```python
from build123d import *

# Parameters (mm, degrees)
BASPROSKE_W        = 5
BASPROSKE_H        = 7
TOOTHCUT_DEPTH     = 12.090536506
TEETHCUTS_COUNT    = 12
TEETHCUTS_ANGLE    = 330
BORSKE_R           = 2.5
BORE_DEPTH         = 50.0000508
SKETCH1_W          = 20.08971131
SKETCH1_H          = 17.337649252
CUT_EXTRUDE3_DEPTH = 0.25


with BuildPart() as part:
    # BasProSke → Base-Revolve (revolve)
    with BuildSketch(Plane(origin=(0, 0, 0), x_dir=(1, 0, 0), z_dir=(0, 1, 0)), mode=Mode.PRIVATE) as base_revolve_sk:
        with Locations((2.5, 3.5)):
            Rectangle(BASPROSKE_W, BASPROSKE_H)
    revolve(base_revolve_sk.sketch.rotate(Axis((-10, 0, 0), (1, 0, 0)), 180), axis=Axis((-10, 0, 0), (1, 0, 0)))

    # TooCutSke → ToothCut (cut, through all)
    with BuildSketch(Plane(origin=(0, 0, 0), x_dir=(0, 0, -1), z_dir=(1, 0, 0))):
        with BuildLine():
            ThreePointArc((0.562207301, 4.715604304), (0, 4.749), (-0.562207301, 4.715604304))
            ThreePointArc((-0.562207301, 4.715604304), (-0.837528627, 5.917009812), (-1.672850686, 6.823328788))
            ThreePointArc((-1.672850686, 6.823328788), (0, 7.0254), (1.672850686, 6.823328788))
            ThreePointArc((1.672850686, 6.823328788), (0.837528627, 5.917009812), (0.562207301, 4.715604304))
        make_face()
    toothcut = extrude(amount=TOOTHCUT_DEPTH, mode=Mode.SUBTRACT)

    # TeethCuts: ToothCut ×12 about axis
    teethcuts_axis = Axis((-10, 0, 0), (1, 0, 0))
    for i in range(1, TEETHCUTS_COUNT):
        add(toothcut.rotate(teethcuts_axis, i * TEETHCUTS_ANGLE / (TEETHCUTS_COUNT - 1)), mode=Mode.SUBTRACT)

    # BorSke → Bore (cut, symmetric)
    with BuildSketch(Plane(origin=(0, 0, 0), x_dir=(0, 0, -1), z_dir=(1, 0, 0))):
        with Locations(Location((0, 0, 0), (0, 0, 180))):
            Circle(BORSKE_R)
    extrude(amount=BORE_DEPTH, both=True, mode=Mode.SUBTRACT)

    # Sketch1 → Cut-Extrude3 (cut)
    with BuildSketch(Plane(origin=(5, 0, 0), x_dir=(0, 0, -1), z_dir=(1, 0, 0))):
        with Locations((2.500843807, -0.387105296)):
            Rectangle(SKETCH1_W, SKETCH1_H)
    extrude(amount=-CUT_EXTRUDE3_DEPTH, mode=Mode.SUBTRACT)


solid = part.part
```
Design review of the part built by this model. Coordinates are the model's own, in mm. A direction names the side the tool comes from. Coordinates: 2 decimals unless noted, no trailing zeros. Write each loop counter-clockwise with the first axis right and the second up, starting at its lowest first coordinate (ties: lowest second). Pieces come first, ordered by that corner, then holes. Notation, with made-up numbers: M -37.75,44.5 L -19.75,44.5 A34 cw -19.75,79.5 Z; hole C 33,10.25 d5. An arc over 180 degrees is marked long. Answer as a JSON object with one key per item and string values.
Item 1: Add section A-A, the plane y = 0. Give the boundary of the cut face in (x, z), and give its area (3 significant figures).
Outcome:
{"outline": "M 0,-4.75 L 4.75,-4.75 L 4.75,-2.5 L 0,-2.5 Z; M 0,2.5 L 4.75,2.5 L 4.75,4.75 L 0,4.75 Z", "area": "21.4 mm²"}
Item 2: Add section C-C, the plane y = 4. Give the boundary of the cut face in (x, z).
Outcome:
{"outline": "M 0,-4.87 L 4.75,-4.87 L 4.75,-2.96 L 0,-2.96 Z; M 0,-2.56 L 4.75,-2.56 L 4.75,2.56 L 0,2.56 Z; M 0,2.96 L 4.75,2.96 L 4.75,4.87 L 0,4.87 Z"}
Item 3: Draft analysis for pull direction Z (two halves, no side actions). For faces 1 (the flat face through (4.75, 0, -3)), 2 (the cylindrical face through (2.342, 5.886, 0.822)), state which applies: pulls with the +Z half, pulls with the -Z half, needs draft (parallel to the pull), parting line crosses it, or undercut.
Outcome:
{"face 1": "needs draft", "face 2": "undercut"}
Item 4: Wall thickness on probe 1 along Z at (x, y) = (0.3, 2); probe 2 along Z at (x, y) = (0.8, -4.25); probe 3 along Y at (x, z) = (1.45, -0.75): over which ranges is each line inside the solid? List them lowest first.
Outcome:
{"probe 1": "-6.67 to -4.6, -4.31 to -1.5, 1.5 to 4.31, 4.6 to 6.67", "probe 2": "-4.97 to -3.15, -2.12 to 2.12, 3.15 to 4.97", "probe 3": "-5.73 to -2.38, 2.38 to 5.73"}
Item 5: Machinability: for faces 3 (the flat face through (0, 0, -3)), 4 (the cylindrical face through (2.342, -4.705, 3.684)), 5 (the cylindrical face through (2.3, -2.4, -4.1)), which of the approach directions +Z, -Z, +X, -X, +Y, -Y give a long, thin tool a straight path to every point of the face, cutting with its end or side? Answer none if there is none.
Outcome:
{"face 3": "+Z, -Z, -X, +Y, -Y", "face 4": "+X, -X, -Y", "face 5": "+X, -X"}
Item 6: Add section D-D, the plane z = 3.25. Give the boundary of the cut face in (x, y), and give its area (3 significant figures).
Outcome:
{"outline": "M 0,-4.36 L 4.75,-4.36 L 4.75,4.36 L 0,4.36 Z", "area": "41.4 mm²"}
Item 7: Insertion check: pin 1 Ø6 at (y, z) = (2, 2) entering from -X; pin 2 Ø2 at (x, y) = (2, 4) entering from -Z. Each pin has a flat end and moves straight along its axis. Give the tip position at first contact, or say it passes through.
Outcome:
{"pin 1": "x = 0", "pin 2": "z = -5.07"}
